Solid Edge part; units mm, degrees
sketch "Sketch1" plane through (0, 0, 0) normal (0, -1, 0) x (1, 0, 0)
  line L0 (-22.5, -22.5) -> (22.5, -22.5)
  line L1 (22.5, -22.5) -> (22.5, 22.5)
  line L2 (22.5, 22.5) -> (-22.5, 22.5)
  line L3 (-22.5, 22.5) -> (-22.5, -22.5)
  dimension "D1" = 22.5
extrude "Protrusion1" add sketch "Sketch1" against normal blind 38
chamfer "Chamfer_1" distance 5 angle 45 4 edges at (22.5, 19, 22.5) (22.5, 19, -22.5) (-22.5, 19, 22.5) (-22.5, 19, -22.5)
hole "Hole1" at (-15.5, 38, 15.5) direction (0, -1, 0) diameter 2.7 end up to next
hole "Hole2" at (-15.5, 38, -15.5) direction (0, -1, 0) diameter 2.7 end up to next
hole "Hole3" at (15.5, 38, -15.5) direction (0, -1, 0) diameter 2.7 end up to next
hole "Hole4" at (15.5, 38, 15.5) direction (0, -1, 0) diameter 2.7 end up to next
sketch "Sketch2" plane through (0, 38, 0) normal (0, 1, 0) x (0, 0, -1)
  circle A0 centre (0, 0) radius 4.35
extrude "Cutout1" cut sketch "Sketch2" against normal up to next
chamfer "Chamfer1" distance 1 angle 45 1 edges at (0, 38, 4.35)
chamfer "Fase_3" distance 1 angle 45 1 edges at (0, 0, 4.35)
chamfer "Fase_5" distance 0.4 angle 45 7 edges at (-15.5, 38, -14.15) (-15.5, 38, 16.85) (15.5, 38, -14.15) (15.5, 38, 16.85) (15.5, 0, 16.85) (15.5, 0, -14.15) (-15.5, 0, -14.15)
sketch "Sketch3" plane through (0, 38, 0) normal (0, 1, 0) x (1, 0, 0)
  circle A0 centre (0, 0) radius 17.5
extrude "Extrusionsausschnitt_2" cut sketch "Sketch3" against normal blind 30
chamfer "Fase_6" distance 1 angle 45 1 edges at (0, 8, 4.35)
properties material "Nylon, allgemein"
Could you check a few things on this model? Use its own coordinates, in mm. A direction names the side the tool comes from. Round coordinates to 2 decimals unless told otherwise and drop trailing zeros. Write each loop counter-clockwise with the first axis right and the second up, starting at its lowest first coordinate (ties: lowest second). Pieces come first, ordered by that corner, then holes. Notation, with made-up numbers: M 69.25,72 L 81.25,72 A11 ccw 81.25,86 Z; hole C 52,-8 d4. An arc over 180 degrees is marked long. Answer in a Markdown table with one row per item. Add a question column.
Q1. Imagine slicing it at C-C (x = 0). Please give me the cut outline in (y, z), then the cut area to 3 significant figures.
Q2. If we mould it in two halves opening along Z, with no side actions, what happens to faces 1 (the flat face through (20, 19, -20)), 2 (the cylindrical face through (16.839, 19.26, 15.324)), 3 (the flat face through (-20, 19, 20))? For each: +Z half, -Z half, draft (parallel to the pull), parting line (faces both ways), or undercut.
Q3. Imagine slicing it at B-B (y = 24.5). Please give me the cut outline in (x, z).
Q4. Imagine slicing it at D-D (z = -15.5). Please give me the cut outline in (x, y), then the cut area to 3 significant figures.
Q5. If I drill on line 1 (Z direction, x = -3, y = 16); line 2 (Z direction, x = 16, y = 23.5); line 3 (Z direction, x = 15, y = 15), over which ranges is the centre line in solid material (lowest first)? Write a range as from..to.
Q6. Will these pins go through, and if not, where does the flat tip stop? pin 1 Ø8 at (x, z) = (10, 3) entering from +Y; pin 2 Ø3 at (x, z) = (-15.5, 15.5) entering from +Y; pin 3 Ø5 at (x, z) = (-12, 2) entering from -Y.
Q7. Imagine slicing it at A-A (z = 0). Please give me the cut outline in (x, y).
Q8. On a 3-axis mill with a long thin cutter (end or side, diameter ignored), from which of +Z, -Z, +X, -X, +Y, -Y can I reach the whole of each face in a straight line? I mean faces 4 (the cylindrical face through (-13.887, 23.21, 10.648)), 5 (the flat face through (-22.5, 19, 0)). Say none if no direction works.
Values:
| question | item | result |
|---|---|---|
| 1 | outline | M 0,-22.5 L 38,-22.5 L 38,-17.5 L 8,-17.5 L 8,-5.35 L 7,-4.35 L 1,-4.35 L 0,-5.35 Z; M 0,5.35 L 1,4.35 L 7,4.35 L 8,5.35 L 8,17.5 L 38,17.5 L 38,22.5 L 0,22.5 Z |
| 1 | area | 588 mm^2 |
| 2 | face 1 | -Z half |
| 2 | face 2 | undercut |
| 2 | face 3 | +Z half |
| 3 | outline | M -22.5,-17.5 L -17.5,-22.5 L 17.5,-22.5 L 22.5,-17.5 L 22.5,17.5 L 17.5,22.5 L -17.5,22.5 L -22.5,17.5 Z; hole C 0,0 d35; hole C -15.5,-15.5 d2.7; hole C -15.5,15.5 d2.7; hole C 15.5,-15.5 d2.7; hole C 15.5,15.5 d2.7 |
| 4 | outline | M -22.5,0 L -17.25,0 L -16.85,0.4 L -16.85,37.6 L -17.25,38 L -22.5,38 Z; M -14.15,0.4 L -13.75,0 L 13.75,0 L 14.15,0.4 L 14.15,37.6 L 13.75,38 L 8.12,38 L 8.12,8 L -8.12,8 L -8.12,38 L -13.75,38 L -14.15,37.6 Z; M 16.85,0.4 L 17.25,0 L 22.5,0 L 22.5,38 L 17.25,38 L 16.85,37.6 Z |
| 4 | area | 1,020 mm^2 |
| 5 | line 1 | -22.5..-17.24, 17.24..22.5 |
| 5 | line 2 | -22.5..-16.75, -14.25..-7.09, 7.09..14.25, 16.75..22.5 |
| 5 | line 3 | -22.5..-16.75, -14.25..-9.01, 9.01..14.25, 16.75..22.5 |
| 6 | pin 1 | y = 8 |
| 6 | pin 2 | y = 37.75 |
| 6 | pin 3 | y = 0 |
| 7 | outline | M -22.5,0 L -5.35,0 L -4.35,1 L -4.35,7 L -5.35,8 L -17.5,8 L -17.5,38 L -22.5,38 Z; M 4.35,1 L 5.35,0 L 22.5,0 L 22.5,38 L 17.5,38 L 17.5,8 L 5.35,8 L 4.35,7 Z |
| 8 | face 4 | +Y |
| 8 | face 5 | +Z, -Z, -X, +Y, -Y |
